from build123d import *

# Parameters (mm, degrees)
F2_R     = 5.08
F4_DEPTH = 2.54
F5_R     = 1.905
F5_W     = 7.62
F5_H     = 2.54
F6_DEPTH = 10.16


with BuildPart() as f1:
    # F0 (on Front) → F1 (revolve)
    with BuildSketch(Plane.XZ):
        Polygon((6.35, 31.75), (0, 0), (12.7, 0), (12.7, 50.8), (0, 50.8), align=None)
    revolve(axis=Axis((12.7, 0, 25.4), (0, 0, -1)))

    # F2
    f2_edges = [f1.edges().sort_by_distance(p)[0] for p in [
        (19.05, 0, 31.75),
        (25.4, 0, 50.8),
    ]]
    fillet(f2_edges, radius=F2_R)

    # F3 (on Front) → F4 (join, symmetric)
    with BuildSketch(Plane.XZ):
        Polygon((10.16, 55.88), (10.16, 50.8), (15.24, 50.8), (15.24, 55.88), (20.32, 55.88), (20.32, 60.96), (15.24, 60.96), (15.24, 66.04), (10.16, 66.04), (10.16, 60.96), (5.08, 60.96), (5.08, 55.88), align=None)
    extrude(amount=F4_DEPTH, both=True)

    # F5 (on Front) → F6 (join)
    with BuildSketch(Plane.XZ):
        with Locations((7.62, 40.3035629486)):
            Circle(F5_R)
        with Locations((17.78, 40.3035629486)):
            Circle(F5_R)
        with Locations((12.7050772909, 36.4935629486)):
            Rectangle(F5_W, F5_H)
    extrude(amount=F6_DEPTH)


solid = f1.part
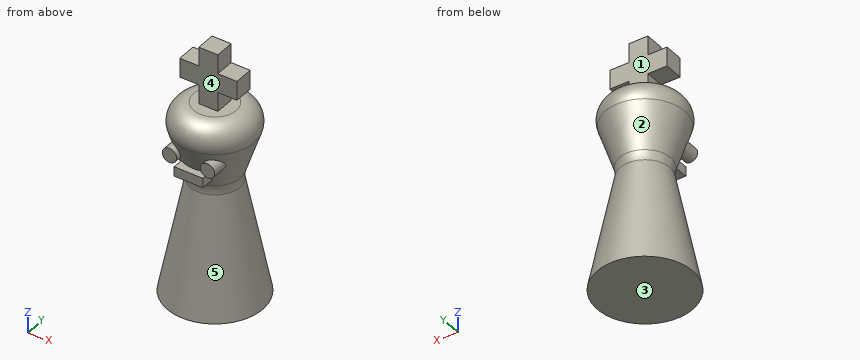
Model file for the job. Use its own axes, mm. Face numbers are marked on the shaded views. A direction names the side the tool comes from. Coordinates: 2 decimals unless noted, no trailing zeros. Loops run counter-clockwise (first coordinate to the right, second up) from the corner with the lowest first, then second, coordinate; pieces in that order, holes last. Notation, with made-up numbers: (50.25, 40) -> (58.25, 40) arc R14 ccw to (58.25, 44) -> close; hole circle Ø9 at (-27, 0.5). An arc over 180 degrees is marked (long way). Use one line per item in the form item = value. Start each with the question number.
(1) Cut at C-C on z = 56.5. Give the cut face in (x, y), and give its area (3 significant figures).
(2) Cut at A-A on z = 25.5. Give the cut face in (x, y), and give its area (3 significant figures).
(3) Probe probe 1 along Z at (x, y) = (9.5, -3); probe 2 along X at (y, z) = (3, 22.5); probe 3 along Y at (x, z) = (17, 59.5). List the from-to ranges inside material, lowest first. Write a range as from..to.
(4) Flat gauge pins, fed straight in: pin 1 (12 mm diameter, centred on x = 10.5, z = 27, fed in from -Y); pin 2 (4 mm diameter, centred on y = 0.5, z = 62.5, fed in from +X); pin 3 (1.5 mm diameter, centred on y = 1, z = 57.5, fed in from -X); pin 4 (1.5 mm diameter, centred on x = 19, y = 3.5, fed in from -Z). Where does each tip first touch, or does it go through?
(5) Tool access for the marked faces 4 and 5: list every direction of +Z, -Z, +X, -X, +Y, -Y with a clear straight run to the whole face (end or side of a thin tool).
(6) Cut at D-D on z = 47. Give the cut face in (x, y).
(7) Pull direction Z, two halves, no side cores. Call the marked faces 1, 2 and 3: pulls with the +Z half, pulls with the -Z half, needs draft (parallel to the pull), parting line crosses it, or undercut.
(8) Cut at B-B on y = -9.5. Give the number of separate pieces and of enclosed holes in the cut face, and give its area (3 significant figures).
Values:
q1.outline = (5.08, -2.54) -> (20.32, -2.54) -> (20.32, 2.54) -> (5.08, 2.54) -> close
q1.area = 77.4 mm2
q2.outline = circle Ø15.2 at (12.7, 0)
q2.area = 181 mm2
q3.probe_1 = 0..50.8
q3.probe_2 = 5.07..20.33
q3.probe_3 = -2.54..2.54
q4.pin_1 = -8.44
q4.pin_2 = 20.32
q4.pin_3 = 5.08
q4.pin_4 = 0
q5.face_4 = +Z, +X, -X, -Y
q5.face_5 = none
q6.outline = circle Ø21.14 at (12.7, 0)
q7.face_1 = needs draft
q7.face_2 = undercut
q7.face_3 = pulls with the -Z half
q8.separate_pieces = 5
q8.enclosed_holes = 0
q8.area = 275 mm2
